```python
from build123d import *

# Parameters (mm, degrees)
BOSS_EXTRUDE1_DEPTH = 1


with BuildPart() as part:
    # Sketch1 → Revolve1 (revolve)
    with BuildSketch(Plane.XY):
        with BuildLine():
            Line((2.2, -4.709624758), (4.85, -6.209624758))
            Line((4.85, -6.209624758), (5, -6.209624758))
            Line((5, -6.209624758), (5, -7.209624758))
            Line((5, -7.209624758), (1.5, -7.209624758))
            Line((1.5, -7.209624758), (1.5, -17.459624758))
            Line((1.5, -17.459624758), (0, -17.459624758))
            Line((0, -17.459624758), (0, 4.709624758))
            ThreePointArc((0, 4.709624758), (4.57123544, 1.133301337), (2.2, -4.164200447))
            ThreePointArc((2.2, -4.164200447), (2.040995641, -4.436912603), (2.2, -4.709624758))
        make_face()
    revolve(axis=Axis((0, 4.709624758, 0), (0, -1, 0)))

    # Sketch3 → Boss-Extrude1 (add)
    with BuildSketch(Plane.XZ.offset(7.209624758)):
        Polygon((5.773502692, 0), (2.886751346, 5), (-2.886751346, 5), (-5.773502692, 0), (-2.886751346, -5), (2.886751346, -5), align=None)
    extrude(amount=-BOSS_EXTRUDE1_DEPTH)


solid = part.part
```
The listing builds one solid part. Answer for the finished solid, in the listing's coordinates (mm). A direction names the side the tool comes from. Coordinates: 2 decimals unless noted, no trailing zeros. Order: outer loops, then holes, each group sorted by start corner. A loop starts at its lowest first (then second) coordinate and runs counter-clockwise, first axis right, second up. Notation, with made-up numbers: M 49,4.25 L 68,4.25 A35 ccw 68,41.25 Z; hole C -9,-7 d6. An arc over 180 degrees is marked long. Answer as a JSON object with one key per item and string values. Group by question number.
1. Section C-C on y = -2.75 is taken. Write down the section's boundary in (x, z).
2. A tool of negligible diameter and unlimited length cuts with its end or side. For faces 4 (the flat face through (1.2, -7.21, 1.2)), 5 (the flat face through (0, -7, 5)), from which of +Z, -Z, +X, -X, +Y, -Y can it reach the whole face along a straight path? Write none if from no direction.
3. Section A-A on x = 0 is taken. Write down the section's boundary in (y, z), then the cut area to 3 significant figures.
4. Straight lines are drawn through the part: line 1 (Y direction, x = 1, z = -2.25); line 2 (Y direction, x = 3, z = 2.5); line 3 (Y direction, x = -2.5, z = -4.25). For each, find the intervals that lie inside material, in ascending order.
5. Determine the mould class of faces 1 (the conical face through (1.092, -4.803, -2.099)), 2 (the flat face through (5, -6.21, -1)), 3 (the flat face through (-4.31, -6.717, 2.535)) for opening direction Y: released by +Y, released by -Y, zero draft, split by the parting line, or undercut.
6. Section B-B on y = -11.75 is taken. Write down the section's boundary in (x, z).
7. Flat-ended cylindrical pins translate along their axes: P1, Ø1, axis at y = 2, z = 2, coming from the +X side; P2, Ø4, axis at y = -1, z = -3.5, coming from the -X side; P3, Ø6, axis at x = 3.5, z = -1, coming from the +Y side. Find the tip coordinate at first contact, or state that the pin passes through.
Values follow:
{
 "1": {"outline": "C 0,0 d7.65"},
 "2": {"face 4": "-Y", "face 5": "+Z, +X, -X, +Y, -Y"},
 "3": {"outline": "M -17.46,-1.5 L -7.21,-1.5 L -7.21,-5 L -6.21,-5 L -6.21,-4.85 L -4.71,-2.2 A0.31 cw -4.16,-2.2 A4.71 ccw long -4.16,2.2 A0.31 cw -4.71,2.2 L -6.21,4.85 L -6.21,5 L -7.21,5 L -7.21,1.5 L -17.46,1.5 Z", "area": "122 mm2"},
 "4": {"line 1": "-7.21 to -4.86, -4.01 to 4.01", "line 2": "-7.21 to -5.67, -2.63 to 2.63", "line 3": "-7.21 to -6.21"},
 "5": {"face 1": "undercut", "face 2": "released by +Y", "face 3": "zero draft"},
 "6": {"outline": "C 0,0 d3"},
 "7": {"P1": "x = 4.09", "P2": "x = -4.41", "P3": "y = 4.67"}
}
